from build123d import *

# Parameters (mm, degrees)
SKETCH1_W           = 30
SKETCH1_H           = 15
BOSS_EXTRUDE1_DEPTH = 7.2
SKETCH2_W           = 5.6
SKETCH2_H           = 5.1
SKETCH2_W_2         = 5.5
SKETCH2_W_3         = 5.4
CUT_EXTRUDE1_DEPTH  = 7.2
SKETCH4_R           = 1.5
CUT_EXTRUDE2_DEPTH  = 7.2
CHAMFER1_SIZE       = 2


with BuildPart() as part:
    # Sketch1 → Boss-Extrude1 (new body)
    with BuildSketch(Plane(origin=(0, 0, 0), x_dir=(1, 0, 0), z_dir=(0, 1, 0))):
        Rectangle(SKETCH1_W, SKETCH1_H)
    extrude(amount=BOSS_EXTRUDE1_DEPTH)

    # Sketch2 → Cut-Extrude1 (cut)
    with BuildSketch(Plane(origin=(0, 7.2, 0), x_dir=(1, 0, 0), z_dir=(0, 1, 0))):
        with Locations((-9, 0)):
            Rectangle(SKETCH2_W, SKETCH2_H)
        Rectangle(SKETCH2_W_2, SKETCH2_H)
        with Locations((10, 0)):
            Rectangle(SKETCH2_W_3, SKETCH2_H)
    extrude(amount=-CUT_EXTRUDE1_DEPTH, mode=Mode.SUBTRACT)

    # Sketch4 → Cut-Extrude2 (cut)
    with BuildSketch(Plane(origin=(0, 0, -7.5), x_dir=(-1, 0, 0), z_dir=(0, 0, -1))):
        with Locations((9, 3.6)):
            Circle(SKETCH4_R)
        with Locations((0, 3.6)):
            Circle(SKETCH4_R)
        with Locations((-10, 3.6)):
            Circle(SKETCH4_R)
    extrude(amount=-CUT_EXTRUDE2_DEPTH, mode=Mode.SUBTRACT)

    # Chamfer1
    chamfer1_edges = [part.edges().sort_by_distance(p)[0] for p in [
        (-15, 3.6, -7.5),
    ]]
    chamfer(chamfer1_edges, length=CHAMFER1_SIZE)


solid = part.part
Work out the finished part from the listing and answer in its coordinate system (mm). A direction names the side the tool comes from. Coordinates: 2 decimals unless noted, no trailing zeros. Write each loop counter-clockwise with the first axis right and the second up, starting at its lowest first coordinate (ties: lowest second). Pieces come first, ordered by that corner, then holes. Notation, with made-up numbers: M -29.5,35 L -14.5,35 A9 ccw -14.5,48 Z; hole C -27,54.25 d2. An arc over 180 degrees is marked long. Write item = value, one per line.
1. The part is cut by section D-D (z = -4). Determine the outline of the cut face in (x, y).
Solution:
outline = M -15,0 L 15,0 L 15,7.2 L -15,7.2 Z; hole C -9,3.6 d3; hole C 0,3.6 d3; hole C 10,3.6 d3
2. Determine the mould class of faces 4 (the face through (0.325, 2.136, -5.06)), 5 (the face through (-14, 3.5, -6.5)), 6 (the face through (3, 0, 0)) for opening direction X: released by +X, released by -X, zero draft, split by the parting line, or undercut.
Solution:
face_4 = undercut
face_5 = released by -X
face_6 = zero draft
3. Straight lines are drawn through the part: line 1 (X direction, y = 3, z = -2.5); line 2 (Y direction, x = 0, z = -6.4); line 3 (Z direction, x = -1.25, y = 5.5). For each, find the intervals that lie inside material, in ascending order. Write a range as from..to.
Solution:
line_1 = -15..-11.8, -6.2..-2.75, 2.75..7.3, 12.7..15
line_2 = 0..2.1, 5.1..7.2
line_3 = -7.5..-2.55, 2.55..7.5
4. The part is cut by section A-A (z = -0.75). Determine the outline of the cut face in (x, y), then the cut area to 3 significant figures.
Solution:
outline = M -15,0 L -11.8,0 L -11.8,7.2 L -15,7.2 Z; M -6.2,0 L -2.75,0 L -2.75,7.2 L -6.2,7.2 Z; M 2.75,0 L 7.3,0 L 7.3,7.2 L 2.75,7.2 Z; M 12.7,0 L 15,0 L 15,7.2 L 12.7,7.2 Z
area = 97.2 mm2
5. For faces 1 (the face through (-6.2, 4, 0)), 2 (the face through (-15, 4, 1)), 3 (the face through (11.2, 2.7, -5.1)), determine the directions among +Z, -Z, +X, -X, +Y, -Y from which every point of the face is accessible in a straight line to the end or side of a thin tool.
Solution:
face_1 = +Y, -Y
face_2 = +Z, -Z, -X, +Y, -Y
face_3 = -Z
6. The part is cut by section C-C (y = 0.5). Determine the outline of the cut face in (x, z), then the cut area to 3 significant figures.
Solution:
outline = M -15,-5.5 L -13,-7.5 L 15,-7.5 L 15,7.5 L -15,7.5 Z; hole M -11.8,-2.55 L -6.2,-2.55 L -6.2,2.55 L -11.8,2.55 Z; hole M -2.75,-2.55 L 2.75,-2.55 L 2.75,2.55 L -2.75,2.55 Z; hole M 7.3,-2.55 L 12.7,-2.55 L 12.7,2.55 L 7.3,2.55 Z
area = 364 mm2
7. A flat-ended cylindrical pin translates along its axis: pin 1 (2.5 mm diameter, centred on x = -9, y = 3.6, fed in from -Z). Find the tip coordinate at first contact, or state that the pin passes through.
Solution:
pin_1 = 2.55
8. The part is cut by section B-B (x = -11). Determine the outline of the cut face in (y, z), then the cut area to 3 significant figures.
Solution:
outline = M 0,-7.5 L 7.2,-7.5 L 7.2,-2.55 L 0,-2.55 Z; M 0,2.55 L 7.2,2.55 L 7.2,7.5 L 0,7.5 Z
area = 71.3 mm2
